Design review of the part shown in the three views and the two pictorial views. Dimensions are in mm from the part's minimum x, y and z. A direction names the side the tool comes from. Coordinates: 2 decimals unless noted, no trailing zeros. Order: outer loops, then holes, each group sorted by start corner. A loop starts at its lowest first (then second) coordinate and runs counter-clockwise, first axis right, second up. Notation, with made-up numbers: M 63,12 L 82,12 A20 cw 82,37 Z; hole C 86,82 d6. An arc over 180 degrees is marked long. Use CSV: the item, a comma, the result in double quotes.
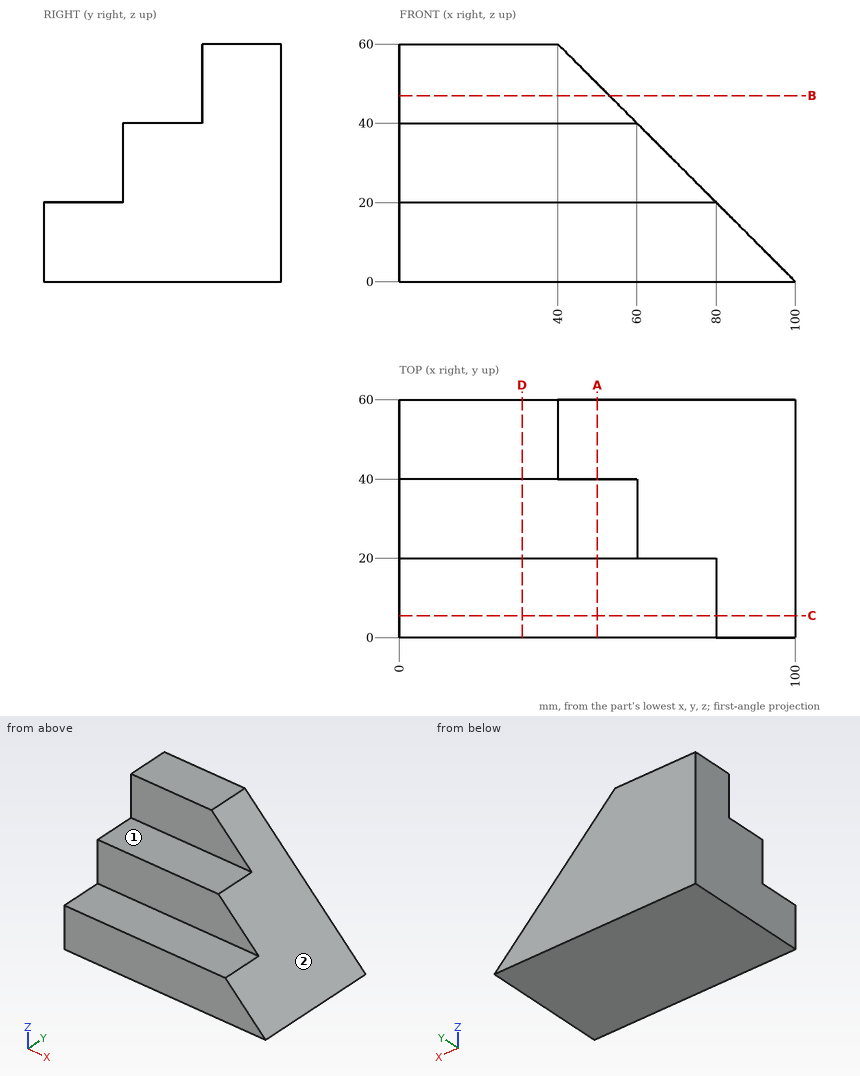
(1) Add section B-B on z = 47. State the section outline as (x, y) points.
The answers:
outline,"M 0,40 L 53,40 L 53,60 L 0,60 Z"
(2) Add section D-D on x = 31. State the section outline as (y, z) points.
The answers:
outline,"M 0,0 L 60,0 L 60,60 L 40,60 L 40,40 L 20,40 L 20,20 L 0,20 Z"
(3) Clearance check with flat-ended pins moving along their axes: P1, Ø6, axis at x = 42.5, y = 27.5, coming from the +Z side; P2, Ø6, axis at y = 33, z = 40.5, coming from the -X side; P3, Ø1, axis at y = 51, z = 31, coming from the +X side; P4, Ø22, axis at x = 40.5, z = 54.5, coming from the -Y side. State where each tip first meets the part, or that it passes through.
The answers:
P1,"stops at z = 40"
P2,"stops at x = 0"
P3,"stops at x = 69.5"
P4,"stops at y = 40"
(4) For the marked faces 1 and 2, list the 3-axis set-ups (+Z, -Z, +X, -X, +Y, -Y) from which the entire face can be reached by the end or side of a thin tool; tool diameter is ignored.
The answers:
face 1,"+Z, +X, -X, -Y"
face 2,"+Z, +X, +Y, -Y"
(5) Wall thickness on probe 1 along Y at (x, z) = (50, 36); probe 2 along Z at (x, y) = (48.5, 31.5); probe 3 along Z at (x, y) = (20, 12): over which ranges is each line inside the solid? List them lowest first.
The answers:
probe 1,"y = 20 to 60"
probe 2,"z = 0 to 40"
probe 3,"z = 0 to 20"
(6) Add section C-C on y = 5.5. State the section outline as (x, z) points, and give its area (3 significant figures).
The answers:
outline,"M 0,0 L 100,0 L 80,20 L 0,20 Z"
area,"1,800 mm2"
(7) Add section A-A on x = 50. State the section outline as (y, z) points, and give its area (3 significant figures).
The answers:
outline,"M 0,0 L 60,0 L 60,50 L 40,50 L 40,40 L 20,40 L 20,20 L 0,20 Z"
area,"2,200 mm2"
